```python
from build123d import *

# Parameters (mm, degrees)
BOSS_EXTRUDE1_DEPTH           = 15
BOSS_EXTRUDE2_REACH           = 38.742
SKETCH3_R                     = 2
SKETCH4_R                     = 3.25
BOSS_EXTRUDE3_DEPTH           = 0.2
FILLET1_R                     = 5
CBORE_FOR_M3_SHCS1_AT_2_COUNT = 2
CBORE_FOR_M3_SHCS1_AT_2_PITCH = 7
SKETCH7_W                     = 5.814312221
SKETCH7_H                     = 13.45156011
BOSS_EXTRUDE4_DEPTH           = 2.5
RIB1_REACH                    = 46.736
SKETCH9_WALL_W                = 96.550792296
SKETCH9_WALL_H                = 8


with BuildPart() as part:
    # Sketch1 → Boss-Extrude1 (new body)
    with BuildSketch(Plane.XY):
        Polygon((0, 0), (0, 15), (5, 15), (15, 28.7), (30, 28.7), (30, 20.7), (17, 20.7), (17, 15), (30, 15), (30, 0), align=None)
    extrude(amount=BOSS_EXTRUDE1_DEPTH)

    # Sketch3 → Boss-Extrude2 (add, up to next)
    with BuildSketch(Plane(origin=(0, 15, 0), x_dir=(1, 0, 0), z_dir=(0, 1, 0)), mode=Mode.PRIVATE) as boss_extrude2_sk1:
        with Locations(Location((25.5, -7.5, 0), (0, 0, 90))):
            Circle(SKETCH3_R)
    boss_extrude2_tool1 = extrude(boss_extrude2_sk1.sketch, amount=BOSS_EXTRUDE2_REACH, mode=Mode.PRIVATE) - part.part
    add(boss_extrude2_tool1.solids().sort_by_distance((25.5, 15, 7.5))[0])

    # Sketch4 → Boss-Extrude3 (add)
    with BuildSketch(Plane(origin=(0, 15, 0), x_dir=(1, 0, 0), z_dir=(0, 1, 0))):
        with Locations(Location((25.5, -7.5, 0), (0, 0, 90))):
            Circle(SKETCH4_R)
    boss_extrude3 = extrude(amount=BOSS_EXTRUDE3_DEPTH)

    # Mirror1: Boss-Extrude3 across plane
    add(boss_extrude3.mirror(Plane.ZX.offset(17.85)))

    # Fillet1
    fillet1_edges = [part.edges().sort_by_distance(p)[0] for p in [
        (0, 7.5, 0),
        (30, 24.7, 0),
        (30, 7.5, 0),
        (30, 24.7, 15),
        (0, 7.5, 15),
        (30, 7.5, 15),
    ]]
    fillet(fillet1_edges, radius=FILLET1_R)

    # Sketch6 → CBORE for M3 SHCS1 (revolve, cut)
    with BuildSketch(Plane(origin=(3, 28.7, 7.5), x_dir=(0, 0, 1), z_dir=(1, 0, 0))):
        Polygon((0, 0), (0, 28.7), (1.7, 28.7), (1.7, 16), (3.25, 16), (3.25, 0.025), (3.275, 0), align=None)
    cbore_for_m3_shcs1 = revolve(axis=Axis((3, 35.05, 7.5), (0, -1, 0)), mode=Mode.SUBTRACT)

    # CBORE for M3 SHCS1 at 2: CBORE for M3 SHCS1 ×2
    with Locations(*[(i * CBORE_FOR_M3_SHCS1_AT_2_PITCH, 0, 0) for i in range(1, CBORE_FOR_M3_SHCS1_AT_2_COUNT)]):
        add(cbore_for_m3_shcs1, mode=Mode.SUBTRACT)

    # Sketch7 → Boss-Extrude4 (add)
    with BuildSketch(Plane(origin=(0, 28.7, 0), x_dir=(1, 0, 0), z_dir=(0, 1, 0))):
        with Locations((30.579754646, -7.5)):
            Rectangle(SKETCH7_W, SKETCH7_H)
    extrude(amount=-BOSS_EXTRUDE4_DEPTH)

    # Sketch9 wall → Rib1 (add, up to next)
    with BuildSketch(Plane(origin=(31.743455378, 24.353734121, 7.5), x_dir=(-0.686573540745, -0.727060364171, 0), z_dir=(0.727060364171, -0.686573540745, 0)), mode=Mode.PRIVATE) as rib1_sk1:
        Rectangle(SKETCH9_WALL_W, SKETCH9_WALL_H)
    rib1_tool1 = extrude(rib1_sk1.sketch, amount=-RIB1_REACH, mode=Mode.PRIVATE) - part.part
    add(rib1_tool1.solids().sort_by_distance((31.743455378, 24.353734121, 7.5))[0])


solid = part.part
```
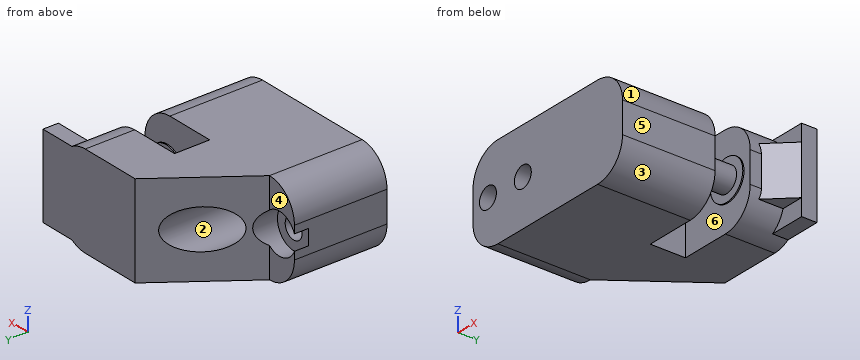
Build history of the part. All positions in model axes, mm. Face numbers are marked on the shaded views. A direction names the side the tool comes from. Give positions to 0.01 mm unless a question says otherwise; leave off trailing zeros. Order: outer loops, then holes, each group sorted by start corner. A loop starts at its lowest first (then second) coordinate and runs counter-clockwise, first axis right, second up. Notation, with made-up numbers: M 82,22.25 L 123,22.25 A20 ccw 123,29.25 Z; hole C 82,27.25 d7. An arc over 180 degrees is marked long. Return JSON: item names as keys, results as strings.
Q1. Flat gauge pins, fed straight in: pin 1 (2 mm diameter, centred on x = 29.5, z = 13.5, fed in from -Y); pin 2 (3 mm diameter, centred on x = 10.5, z = 9, fed in from +Y); pin 3 (2 mm diameter, centred on x = 29, y = 25, fed in from +Z); pin 4 (1.5 mm diameter, centred on y = 6, z = 8.5, fed in from +X). Where does each tip first touch, or does it go through?
Answer list:
{"pin 1": "stops at y = 0", "pin 2": "stops at y = 12.7", "pin 3": "stops at z = 14", "pin 4": "stops at x = 30"}
Q2. Band-saw the part on C-C (z = 13). Give the cut face in (x, y).
Answer list:
{"outline": "M 1,0 L 29,0 L 29,15 L 17,15 L 17,20.7 L 29,20.7 L 29,26.2 L 33.49,26.2 L 33.49,28.7 L 15,28.7 L 5,15 L 1,15 Z"}
Q3. Band-saw the part on B-B (y = 16). Give the cut face in (x, z), then the cut area to 3 significant figures.
Answer list:
{"outline": "M 5.73,0 L 17,0 L 17,15 L 5.73,15 L 5.73,9.26 A3.25 cw 5.73,5.74 Z; C 25.5,7.5 d4; hole C 10,7.5 d6.5", "area": "147 mm^2"}
Q4. 3-axis set-ups, long thin cutter, end or side, ignore diameter. For the marked faces 4, 5 and 6: which of +Z, -Z, +X, -X, +Y, -Y reach the whole face in a straight line?
Answer list:
{"face 4": "+Z, -Z, -X, +Y", "face 5": "+Z, -Z, +X, -Y", "face 6": "none"}
Q5. Band-saw the part on D-D (y = 19.25). Give the cut face in (x, z).
Answer list:
{"outline": "M 8.1,0 L 17,0 L 17,15 L 8.1,15 L 8.1,10.14 A3.25 cw long 8.1,4.86 Z; C 25.5,7.5 d4"}
Q6. Band-saw the part on A-A (x = 19). Give the cut face in (y, z), then the cut area to 3 significant figures.
Answer list:
{"outline": "M 0,0 L 15,0 L 15,15 L 0,15 Z; M 20.7,0 L 28.7,0 L 28.7,15 L 20.7,15 Z", "area": "345 mm^2"}
Q7. Wall check: probe 1 along X at (y, z) = (5.75, 7.5); probe 2 along Y at (x, z) = (27, 11.5); probe 3 along Z at (x, y) = (10, 17). Give the ranges that are in metal, low to high. Write a range as from..to.
Answer list:
{"probe 1": "x = 0..1.3, 4.7..8.3, 11.7..30", "probe 2": "y = 0..15, 20.7..28.7", "probe 3": "z = 0..4.25, 10.75..15"}
Q8. Two-plate mould, pull along Z, no slides. Class the marked faces 1, 2 and 3: pulls with the +Z half, pulls with the -Z half, needs draft (parallel to the pull), parting line crosses it, or undercut.
Answer list:
{"face 1": "pulls with the +Z half", "face 2": "undercut", "face 3": "pulls with the -Z half"}
